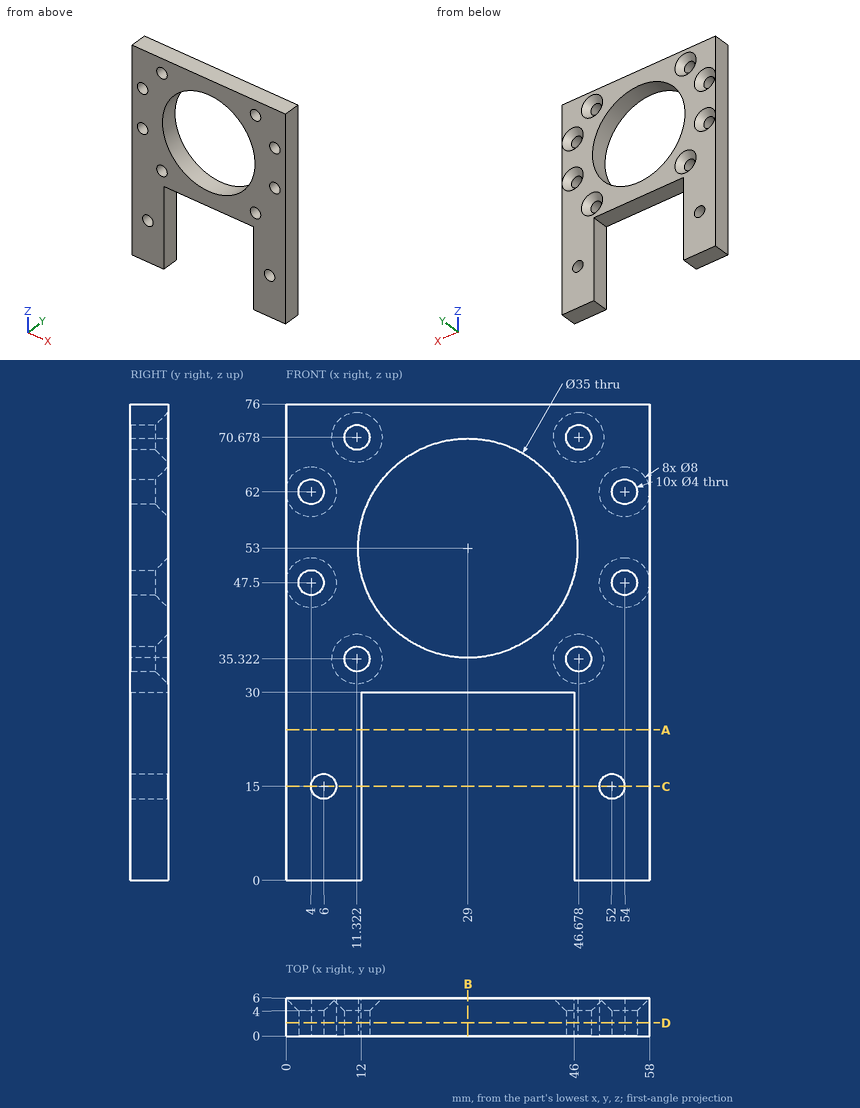
Geometry: see drawing. Coordinates: mm, zero at the bounding-box minimum. Round coordinates to 2 decimals unless told otherwise and drop trailing zeros. Loops run counter-clockwise (first coordinate to the right, second up) from the corner with the lowest first, then second, coordinate; pieces in that order, holes last.
(1) Section query A-A (z = 24). Output: boundary loops of the cut face in (x, y).
From the geometry:
outline: (0, 0) - (12, 0) - (12, 6) - (0, 6) - close; (46, 0) - (58, 0) - (58, 6) - (46, 6) - close
(2) Contact query for a flat-ended pin moving along its axis: pin 1 Ø5 at (x, z) = (11.32, 35.32) entering from +Y. Output: stop coordinate, or through.
From the geometry:
pin 1: stops at y = 4.5
(3) Material intervals for probe 1 along X at (y, z) = (3.7, 9); probe 2 along Z at (x, y) = (3.5, 1.95); probe 3 along X at (y, z) = (3.1, 47.5), sorted ascending.
From the geometry:
probe 1: x = 0 to 12, 46 to 58
probe 2: z = 0 to 45.56, 49.44 to 60.06, 63.94 to 76
probe 3: x = 0 to 2, 6 to 12.39, 45.61 to 52, 56 to 58
(4) Section query B-B (x = 29). Output: boundary loops of the cut face in (y, z).
From the geometry:
outline: (0, 30) - (6, 30) - (6, 35.5) - (0, 35.5) - close; (0, 70.5) - (6, 70.5) - (6, 76) - (0, 76) - close
(5) Section query C-C (z = 15). Output: boundary loops of the cut face in (x, y).
From the geometry:
outline: (0, 0) - (4, 0) - (4, 6) - (0, 6) - close; (8, 0) - (12, 0) - (12, 6) - (8, 6) - close; (46, 0) - (50, 0) - (50, 6) - (46, 6) - close; (54, 0) - (58, 0) - (58, 6) - (54, 6) - close
(6) Section query D-D (y = 2.1). Give the number of separate pieces and of enclosed holes in the cut face, and give its area (3 significant figures).
From the geometry:
separate pieces: 1
enclosed holes: 11
area: 2,300 mm2
